from build123d import *

# Parameters (mm, degrees)
SKETCH1_W           = 50.8
SKETCH1_H           = 81.28
BOSS_EXTRUDE1_DEPTH = 0.8001
SKETCH2_R           = 1.5875
CUT_EXTRUDE1_DEPTH  = 48.951331994
FILLET1_R           = 3.175


with BuildPart() as part:
    # Sketch1 → Boss-Extrude1 (new, symmetric)
    with BuildSketch(Plane(origin=(0, 0, 0), x_dir=(1, 0, 0), z_dir=(0, 1, 0))):
        Rectangle(SKETCH1_W, SKETCH1_H)
    extrude(amount=BOSS_EXTRUDE1_DEPTH, both=True)

    # Sketch2 → Cut-Extrude1 (cut, through all)
    with BuildSketch(Plane(origin=(0, 0.8001, 0), x_dir=(1, 0, 0), z_dir=(0, 1, 0))):
        with Locations(Location((0, 36.83, 0), (0, 0, 270))):
            Circle(SKETCH2_R)
        with Locations(Location((0, -36.83, 0), (0, 0, 270))):
            Circle(SKETCH2_R)
    extrude(amount=-CUT_EXTRUDE1_DEPTH, mode=Mode.SUBTRACT)

    # Fillet1
    fillet1_edges = [part.edges().sort_by_distance(p)[0] for p in [
        (25.4, 0, 40.64),
        (-25.4, 0, 40.64),
        (-25.4, 0, -40.64),
        (25.4, 0, -40.64),
    ]]
    fillet(fillet1_edges, radius=FILLET1_R)


solid = part.part
Input: part model. Units: mm. Frame: model coordinates. Coordinates: 2 decimals unless noted, no trailing zeros. Loops run counter-clockwise (first coordinate to the right, second up) from the corner with the lowest first, then second, coordinate; pieces in that order, holes last.
Q1. Contact query for a flat-ended pin moving along its axis: pin 1 (2.5 mm diameter, centred on x = 0, z = 36.83, fed in from -Y). Output: stop coordinate, or through.
Q2. Material intervals for line 1 (X direction, y = 0.25, z = 36.83); line 2 (Z direction, x = 22.5, y = -0.05), sorted ascending.
Q3. Draft query along X for faces 1 (the face through (0.07, 0.011, 35.244)), 2 (the face through (0.477, 0.011, -35.316)), 3 (the face through (-25.4, 0, 1)), 4 (the face through (0, -0.8, -1)). Return one class per face: +X half, -X half, draft (parallel to the pull), parting line (faces both ways), or undercut.
Q4. Cut plane A-A (x = 0). Output: boundary loops of the cut face in (y, z), then the cut area to 3 significant figures.
Working result:
1. pin 1: passes through
2. line 1: x = -25.4 to -1.59, 1.59 to 25.4
2. line 2: z = -40.63 to 40.63
3. face 1: undercut
3. face 2: undercut
3. face 3: -X half
3. face 4: draft
4. outline: (-0.8, -40.64) - (0.8, -40.64) - (0.8, -38.42) - (-0.8, -38.42) - close; (-0.8, -35.24) - (0.8, -35.24) - (0.8, 35.24) - (-0.8, 35.24) - close; (-0.8, 38.42) - (0.8, 38.42) - (0.8, 40.64) - (-0.8, 40.64) - close
4. area: 120 mm2
